The model under review builds one solid part; all positions refer to its coordinate system, in mm. Round coordinates to 2 decimals unless told otherwise and drop trailing zeros. Write each loop counter-clockwise with the first axis right and the second up, starting at its lowest first coordinate (ties: lowest second). Pieces come first, ordered by that corner, then holes. Notation, with made-up numbers: M -18,-29 L 21,-29 A26 cw 21,-1 Z; hole C 83,-12.75 d8. An arc over 180 degrees is marked long. Write item = value, one per line. Start each with the question number.
Item 1: Take a section at C-C, the plane x = -15.5. Give the boundary of the cut face in (y, z) (3 decimals).
Item 2: Take a section at A-A, the plane z = 6.25. Give the boundary of the cut face in (x, y) (3 decimals).
Item 3: Take a section at B-B, the plane y = 15. Give the boundary of the cut face in (x, z) (3 decimals).
Item 4: To check wall thickness, follow line 1 along X through (y, z) = (-15.5, 1.75) (3 decimals); line 2 along X through (y, z) = (-15, 4) (3 decimals). State the ranges of each line that lie inside material, in increasing order.
Item 5: For pin 1 Ø2.5 at (x, y) = (-15.5, -15.5) entering from -Z; pin 2 Ø3.5 at (x, y) = (15.5, -15.5) entering from -Z, all flat-tipped, find the tip position at first contact; note any pin that passes through.
Item 6: The part is to be moulded in two halves that separate along X. For faces 1 (the flat face through (-21, 0, 3)), 2 (the cylindrical face through (-14, -15.57, 3.55)), 3 (the flat face through (0, -21, 3)), say which applies: +X half, -X half, draft (parallel to the pull), parting line (faces both ways), or undercut.
from build123d import *

# Parameters (mm, degrees)
F0_W     = 42
F0_H     = 42
F1_DEPTH = 7
F2_SIZE  = 7.325
F3_D     = 3


with BuildPart() as f1:
    # F0 (on Top) → F1 (new body)
    with BuildSketch(Plane.XY):
        Rectangle(F0_W, F0_H)
    extrude(amount=F1_DEPTH)

    # F2
    f2_edges = [f1.edges().sort_by_distance(p)[0] for p in [
        (-21, -21, 3.5),
        (21, -21, 3.5),
        (21, 21, 3.5),
        (-21, 21, 3.5),
    ]]
    chamfer(f2_edges, length=F2_SIZE)

    # F3 (through all)
    with Locations(Plane(origin=(0, 0, 0), x_dir=(1, 0, 0), z_dir=(0, 0, -1))):
        with Locations((15.5, 15.5), (-15.5, 15.5), (-15.5, -15.5), (15.5, -15.5)):
            Hole(F3_D / 2)


solid = f1.part
Response values:
q1.outline = M -19.175,0 L -17,0 L -17,7 L -19.175,7 Z; M -14,0 L 14,0 L 14,7 L -14,7 Z; M 17,0 L 19.175,0 L 19.175,7 L 17,7 Z
q2.outline = M -21,-13.675 L -13.675,-21 L 13.675,-21 L 21,-13.675 L 21,13.675 L 13.675,21 L -13.675,21 L -21,13.675 Z; hole C -15.5,-15.5 d3; hole C -15.5,15.5 d3; hole C 15.5,-15.5 d3; hole C 15.5,15.5 d3
q3.outline = M -19.675,0 L -16.914,0 L -16.914,7 L -19.675,7 Z; M -14.086,0 L 14.086,0 L 14.086,7 L -14.086,7 Z; M 16.914,0 L 19.675,0 L 19.675,7 L 16.914,7 Z
q4.line_1 = -19.175 to -17, -14 to 14, 17 to 19.175
q4.line_2 = -19.675 to -16.914, -14.086 to 14.086, 16.914 to 19.675
q5.pin_1 = through
q5.pin_2 = 0
q6.face_1 = -X half
q6.face_2 = undercut
q6.face_3 = draft
